Could you check a few things on this drawing? It's one solid part, dimensions in mm from its lowest x, y, z. Round coordinates to 2 decimals unless told otherwise and drop trailing zeros. Loops run counter-clockwise (first coordinate to the right, second up) from the corner with the lowest first, then second, coordinate; pieces in that order, holes last. Notation, with made-up numbers: (-22, -28) -> (-16, -28) arc R24 cw to (-16, 9) -> close; hole circle Ø10 at (23.25, -19.75). An arc over 180 degrees is marked (long way). Use one line per item in the form item = value. Start each with the question number.
Item 1: If I drill on L1, parallel to X at y = 1.35, z = 5; L2, parallel to Z at x = 47.5, y = 2.2; L3, parallel to Z at x = 30.5, y = 0.5, over which ranges is the centre line in solid material (lowest first)? Write a range as [from, to].
Item 2: If we section it at C-C (z = 5): Write out the boundary of the cut face in (x, y).
Item 3: If we section it at A-A (x = 47.5): Write out the boundary of the cut face in (y, z).
Item 4: If we section it at B-B (y = 2.3): Write out the boundary of the cut face in (x, z).
Item 5: I'm going to push a flat-ended pin straight in: pin 1 Ø2 at (x, z) = (83, 8.5) entering from -Y. Where does the tip first touch, or does it pass through?
Item 6: If we section it at D-D (x = 15): Write out the boundary of the cut face in (y, z), then the cut area to 3 significant figures.
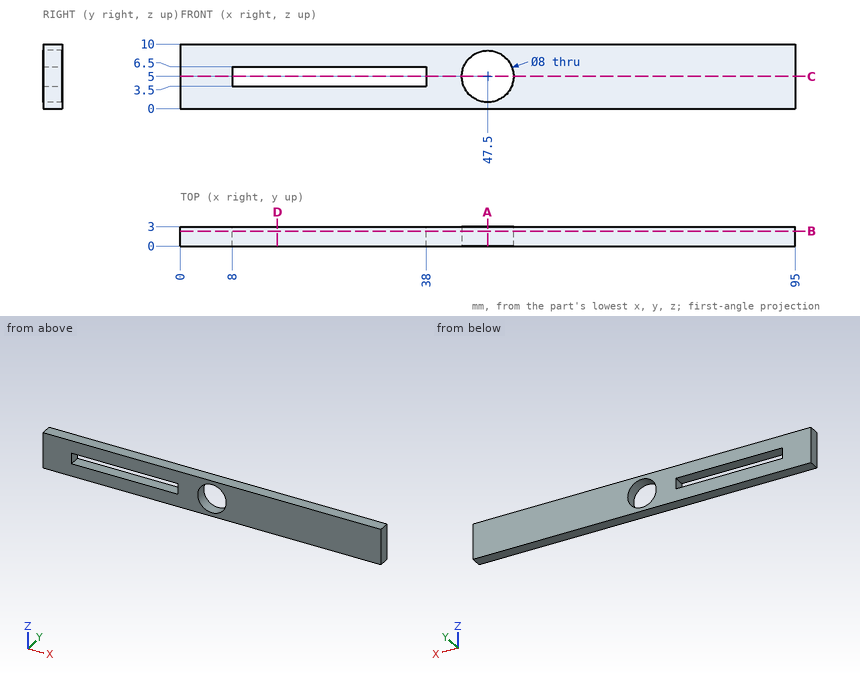
Values found:
q1.L1 = [0, 8], [38, 43.5], [51.5, 95]
q1.L2 = [0, 1], [9, 10]
q1.L3 = [0, 3.5], [6.5, 10]
q2.outline = (0, 0) -> (8, 0) -> (8, 3) -> (0, 3) -> close; (38, 0) -> (43.5, 0) -> (43.5, 3) -> (38, 3) -> close; (51.5, 0) -> (95, 0) -> (95, 3) -> (51.5, 3) -> close
q3.outline = (0, 0) -> (3, 0) -> (3, 1) -> (0, 1) -> close; (0, 9) -> (3, 9) -> (3, 10) -> (0, 10) -> close
q4.outline = (0, 0) -> (95, 0) -> (95, 10) -> (0, 10) -> close; hole (8, 3.5) -> (38, 3.5) -> (38, 6.5) -> (8, 6.5) -> close; hole circle Ø8 at (47.5, 5)
q5.pin_1 = 0
q6.outline = (0, 0) -> (3, 0) -> (3, 3.5) -> (0, 3.5) -> close; (0, 6.5) -> (3, 6.5) -> (3, 10) -> (0, 10) -> close
q6.area = 21.0 mm2
